Part model, mm, in its own coordinate system. Face numbers are marked on the shaded views. Give positions to 0.01 mm unless a question says otherwise; leave off trailing zeros. Loops run counter-clockwise (first coordinate to the right, second up) from the corner with the lowest first, then second, coordinate; pieces in that order, holes last. Notation, with made-up numbers: (14.5, 20) -> (28.5, 20) arc R12 ccw to (28.5, 32) -> close; hole circle Ø9 at (-27.5, 12). An arc over 180 degrees is marked (long way). One line per question, with ' | ' between items.
```python
from build123d import *

# Parameters (mm, degrees)
SKETCH1_R           = 3.75
SKETCH1_R_2         = 1.25
BOSS_EXTRUDE1_DEPTH = 5
CUT_EXTRUDE1_DEPTH  = 8.288689869
CIRPATTERN1_COUNT   = 23


with BuildPart() as part:
    # Sketch1 → Boss-Extrude1 (new body)
    with BuildSketch(Plane.XY):
        Circle(SKETCH1_R)
        Circle(SKETCH1_R_2, mode=Mode.SUBTRACT)
    extrude(amount=BOSS_EXTRUDE1_DEPTH)

    # Sketch2 → Cut-Extrude1 (cut, through all)
    with BuildSketch(Plane.XY):
        Polygon((0, 3.211260138), (1.027348171, 4.238608309), (-1.027348171, 4.238608309), align=None)
    cut_extrude1 = extrude(amount=CUT_EXTRUDE1_DEPTH, mode=Mode.SUBTRACT)

    # CirPattern1: Cut-Extrude1 ×23 about axis
    cirpattern1_axis = Axis((0, 0, 0), (0, 0, 1))
    for i in range(1, CIRPATTERN1_COUNT):
        add(cut_extrude1.rotate(cirpattern1_axis, i * 360 / CIRPATTERN1_COUNT), mode=Mode.SUBTRACT)


solid = part.part
```
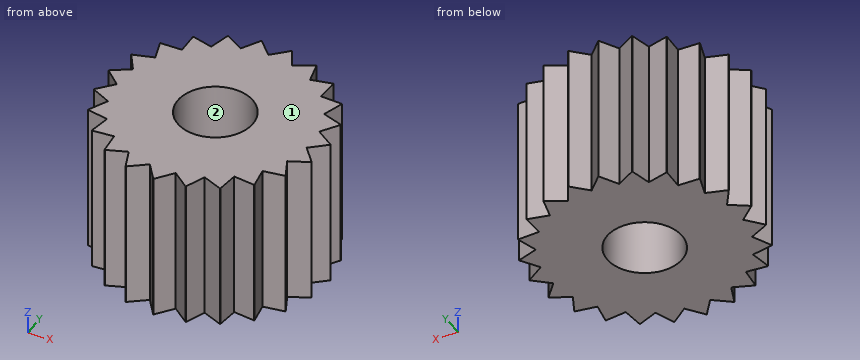
1) Pin check, flat tips, straight feed: P1, Ø1.5, axis at x = 1.5, z = 4.5, coming from the +Y side; P2, Ø2, axis at x = 0, y = 0, coming from the -Z side. Stop position of each tip, or through.
Found:
P1: y = 3.44 | P2: through
2) Drill centre lines: line 1 (X direction, y = 0.5, z = 2.8); line 2 (Y direction, x = 0.25, z = 3.9); line 3 (X direction, y = -0.25, z = 3.4). Where is each one in solid material? Low to high.
Found:
line 1: -3.38 to -1.15, 1.15 to 3.38 | line 2: -3.43 to -1.22, 1.22 to 3.46 | line 3: -3.23 to -1.22, 1.22 to 3.23
3) Saw through at B-B (x = -0.25). Give the cut face in (y, z).
Found:
outline: (-3.43, 0) -> (-1.22, 0) -> (-1.22, 5) -> (-3.43, 5) -> close; (1.22, 0) -> (3.46, 0) -> (3.46, 5) -> (1.22, 5) -> close
4) Saw through at A-A (y = 0). Give the cut face in (x, z), and give its area (3 significant figures).
Found:
outline: (-3.46, 0) -> (-1.25, 0) -> (-1.25, 5) -> (-3.46, 5) -> close; (1.25, 0) -> (3.46, 0) -> (3.46, 5) -> (1.25, 5) -> close | area: 22.1 mm2
5) Saw through at D-D (x = -2.5). Give the cut face in (y, z).
Found:
outline: (-2.54, 0) -> (2.19, 0) -> (2.19, 5) -> (-2.54, 5) -> close
6) Pull direction Y, two halves, no side cores. Call the marked faces 1 and 2: pulls with the +Y half, pulls with the -Y half, needs draft (parallel to the pull), parting line crosses it, or undercut.
Found:
face 1: needs draft | face 2: undercut
7) Saw through at C-C (y = 2.5). Give the cut face in (x, z).
Found:
outline: (-2.36, 0) -> (2.36, 0) -> (2.36, 5) -> (-2.36, 5) -> close
